Here's how the part is built. I have some questions about the finished solid (model axes, mm). Face numbers are marked on the shaded views. Give positions to 0.01 mm unless a question says otherwise; leave off trailing zeros. Write each loop counter-clockwise with the first axis right and the second up, starting at its lowest first coordinate (ties: lowest second). Pieces come first, ordered by that corner, then holes. Notation, with made-up numbers: (-25.5, 16) -> (31.5, 16) arc R16 ccw to (31.5, 47) -> close; hole circle Ø11 at (-7, 40.25). An arc over 180 degrees is marked (long way). Use CSV: the item, a comma, the result in double quotes. Start each with the question number.
(1) Suppose I cut it at B-B on z = 5.05. List the corners of the cut face in (x, y) for me.
(2) For pin 1 Ø1 at (x, z) = (7, 1.5) entering from +Y; pin 2 Ø1.6 at (x, z) = (16.5, 1.5) entering from +Y; pin 3 Ø1.5 at (x, z) = (7.5, 2.5) entering from +Y; pin 4 Ø1.8 at (x, y) = (10, 12) entering from -Z, each with a flat end and sliding along its axis, tell me the tip position at first contact or that it passes through.
(3) Suppose I cut it at A-A on y = 12. List the corners of the cut face in (x, z) for me, plus the area to 3 significant figures.
(4) Suppose I cut it at D-D on y = 42.5. List the corners of the cut face in (x, z) for me.
(5) If we mould it in two halves opening along Y, with no side actions, what happens to the marked faces 1 and 2? For each: pulls with the +Y half, pulls with the -Y half, needs draft (parallel to the pull), parting line crosses it, or undercut.
(6) Suppose I cut it at C-C on x = 10. Give the number of separate pieces and of enclosed holes in the cut face, plus the area to 3 significant figures.
(7) I need wall thicknesses on L1, parallel to Y at x = 10, z = 4.4; L2, parallel to Y at x = 10, z = 1.65; L3, parallel to Y at x = 10, z = 1.45. Which ranges of each line are inside material? Lowest first, please. Write a range as [from, to].
from build123d import *

# Parameters (mm, degrees)
SKETCH_R        = 1.65
SKETCH_R_2      = 1.1
SKETCH_W        = 2.2
SKETCH_H        = 2.2
PAD_DEPTH       = 2
CHAMFER_SIZE    = 1.65
SKETCH001_R     = 4
SKETCH001_R_2   = 1.65
PAD001_DEPTH    = 4
CHAMFER001_SIZE = 1.2


with BuildPart() as chamfer_body:
    # Sketch → Pad (new body)
    with BuildSketch(Plane.XY):
        with BuildLine():
            Line((0, 10), (0, 64))
            ThreePointArc((20, 64), (10, 74), (0, 64))
            Line((20, 64), (20, 10))
            ThreePointArc((0, 10), (10, 0), (20, 10))
        make_face()
        with Locations((10, 69)):
            Circle(SKETCH_R, mode=Mode.SUBTRACT)
        with Locations((10, 5)):
            Circle(SKETCH_R, mode=Mode.SUBTRACT)
        with Locations((10, 62)):
            Circle(SKETCH_R_2, mode=Mode.SUBTRACT)
        with Locations((10, 12)):
            Circle(SKETCH_R_2, mode=Mode.SUBTRACT)
        with Locations((3.75, 39.5)):
            Rectangle(SKETCH_W, SKETCH_H, mode=Mode.SUBTRACT)
        with Locations((3.75, 37)):
            Rectangle(SKETCH_W, SKETCH_H, mode=Mode.SUBTRACT)
        with Locations((3.75, 34.5)):
            Rectangle(SKETCH_W, SKETCH_H, mode=Mode.SUBTRACT)
        with Locations((6.25, 34.5)):
            Rectangle(SKETCH_W, SKETCH_H, mode=Mode.SUBTRACT)
        with Locations((6.25, 37)):
            Rectangle(SKETCH_W, SKETCH_H, mode=Mode.SUBTRACT)
        with Locations((6.25, 39.5)):
            Rectangle(SKETCH_W, SKETCH_H, mode=Mode.SUBTRACT)
        with Locations((13.75, 39.5)):
            Rectangle(SKETCH_W, SKETCH_H, mode=Mode.SUBTRACT)
        with Locations((13.75, 37)):
            Rectangle(SKETCH_W, SKETCH_H, mode=Mode.SUBTRACT)
        with Locations((13.75, 34.5)):
            Rectangle(SKETCH_W, SKETCH_H, mode=Mode.SUBTRACT)
        with Locations((16.25, 34.5)):
            Rectangle(SKETCH_W, SKETCH_H, mode=Mode.SUBTRACT)
        with Locations((16.25, 37)):
            Rectangle(SKETCH_W, SKETCH_H, mode=Mode.SUBTRACT)
        with Locations((16.25, 39.5)):
            Rectangle(SKETCH_W, SKETCH_H, mode=Mode.SUBTRACT)
    extrude(amount=PAD_DEPTH)

    # Chamfer
    chamfer_edges = [chamfer_body.edges().sort_by_distance(p)[0] for p in [
        (8.35, 69, 0),
        (8.35, 5, 0),
    ]]
    chamfer(chamfer_edges, length=CHAMFER_SIZE)


with BuildPart() as chamfer001:
    # Sketch001 → Pad001 (new body)
    with BuildSketch(Plane.XY.offset(2)):
        with Locations((10, 69)):
            Circle(SKETCH001_R)
        with Locations((10, 69)):
            Circle(SKETCH001_R_2, mode=Mode.SUBTRACT)
        with Locations((10, 5)):
            Circle(SKETCH001_R)
        with Locations((10, 5)):
            Circle(SKETCH001_R_2, mode=Mode.SUBTRACT)
    extrude(amount=PAD001_DEPTH)

    # Fusion: union Chamfer body
    add(chamfer_body.part)

    # Chamfer001
    chamfer001_edges = [chamfer001.edges().sort_by_distance(p)[0] for p in [
        (8.9, 62, 0),
        (8.9, 12, 0),
    ]]
    chamfer(chamfer001_edges, length=CHAMFER001_SIZE)


solid = chamfer001.part
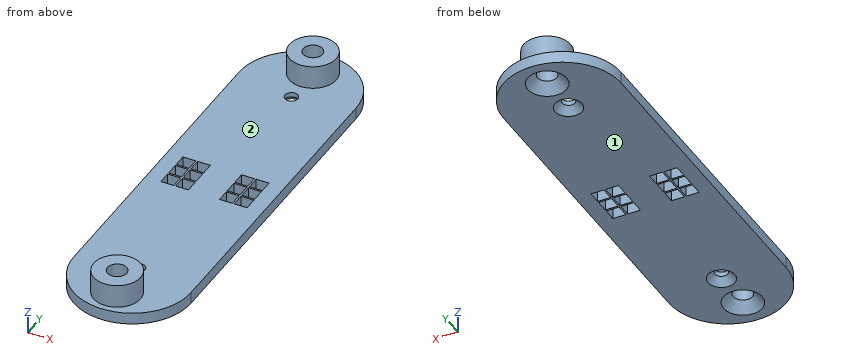
Geometry says:
1,outline,"circle Ø8 at (10, 5); circle Ø8 at (10, 69); hole circle Ø3.3 at (10, 5); hole circle Ø3.3 at (10, 69)"
2,pin 1,"y = 73.68"
2,pin 2,"y = 72.22"
2,pin 3,"y = 73.81"
2,pin 4,"through"
3,outline,"(0, 0) -> (7.7, 0) -> (8.9, 1.2) -> (8.9, 2) -> (0, 2) -> close; (11.1, 1.2) -> (12.3, 0) -> (20, 0) -> (20, 2) -> (11.1, 2) -> close"
3,area,"34.2 mm²"
4,outline,"(0, 0) -> (20, 0) -> (20, 2) -> (0, 2) -> close"
5,face 1,"needs draft"
5,face 2,"undercut"
6,separate pieces,"5"
6,enclosed holes,"0"
6,area,"155 mm²"
7,L1,"[1, 3.35], [6.65, 9], [65, 67.35], [70.65, 73]"
7,L2,"[0, 3.35], [6.65, 10.9], [13.1, 60.9], [63.1, 67.35], [70.65, 74]"
7,L3,"[0, 3.15], [6.85, 10.9], [13.1, 60.9], [63.1, 67.15], [70.85, 74]"
